Source: three-view drawing plus pictorial views. Frame: mm from the lowest corner of the part. A direction names the side the tool comes from. Round coordinates to 2 decimals unless told otherwise and drop trailing zeros. Order: outer loops, then holes, each group sorted by start corner. A loop starts at its lowest first (then second) coordinate and runs counter-clockwise, first axis right, second up. Notation, with made-up numbers: (28, -23.5) -> (47, -23.5) arc R28 cw to (47, 10.5) -> close; hole circle Ø2 at (-38.75, 33.25). An arc over 180 degrees is marked (long way). Answer as CSV lines item,"result".
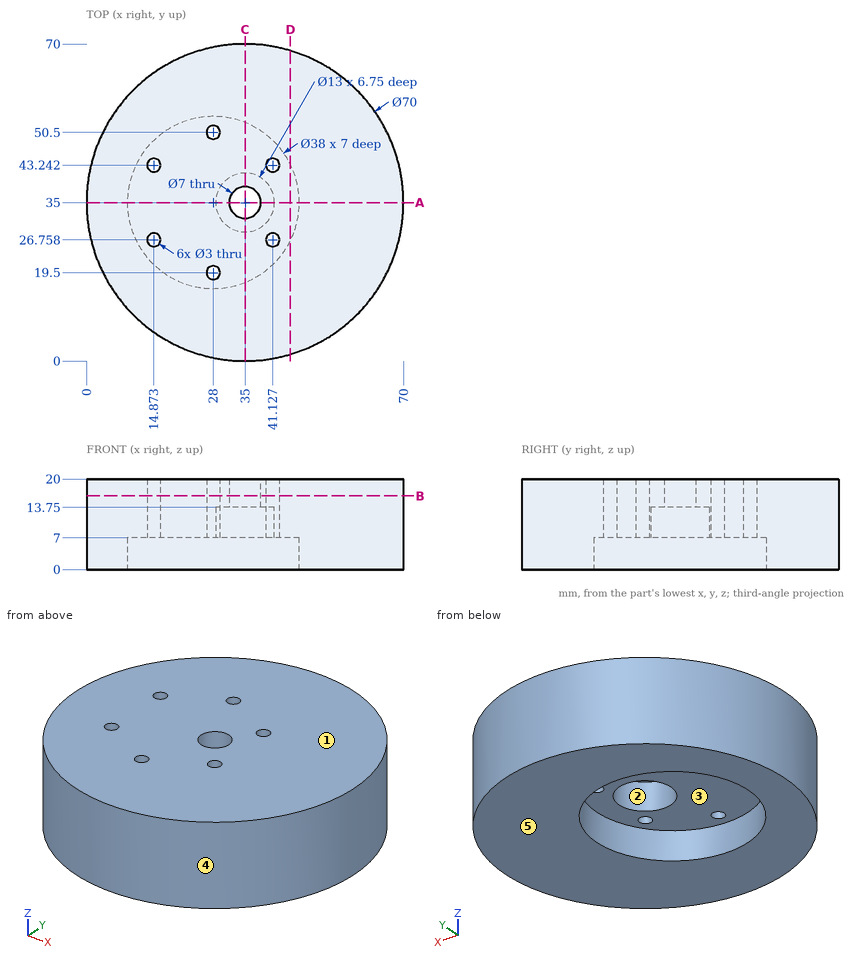
1. Pin query (flat end, axial travel): pin 1 (1.8 mm diameter, centred on x = 41.13, y = 43.24, fed in from -Z); pin 2 (1.5 mm diameter, centred on y = 43, z = 3, fed in from +X); pin 3 (12 mm diameter, centred on x = 48, z = 4, fed in from +Y); pin 4 (4 mm diameter, centred on y = 54.5, z = 5, fed in from -X). Return the tip coordinate at first contact, or that it passes through.
Results below:
pin 1,"through"
pin 2,"x = 69.24"
pin 3,"y = 69.29"
pin 4,"x = 4.69"
2. Section query D-D on x = 45. Return loops of the section in (y, z).
Results below:
outline,"(1.46, 0) -> (26.51, 0) -> (26.51, 7) -> (43.49, 7) -> (43.49, 0) -> (68.54, 0) -> (68.54, 20) -> (1.46, 20) -> close"
3. Line query: L1, parallel to Y at x = 28, z = 17; L2, parallel to Z at x = 35.5, y = 40; L3, parallel to Y at x = 41, z = 5.5. Output: solid intervals per line, ascending. Write a range as [from, to].
Results below:
L1,"[0.71, 18], [21, 49], [52, 69.29]"
L2,"[13.75, 20]"
L3,"[0.52, 21.14], [48.86, 69.48]"
4. Reachability of the marked faces 1 and 2 from +Z, -Z, +X, -X, +Y, -Y: full face, straight path, thin tool, end or side. Return the list, or none.
Results below:
face 1,"+Z, +X, -X, +Y, -Y"
face 2,"-Z"
5. Section query C-C on x = 35. Return loops of the section in (y, z).
Results below:
outline,"(0, 0) -> (17.34, 0) -> (17.34, 7) -> (28.5, 7) -> (28.5, 13.75) -> (31.5, 13.75) -> (31.5, 20) -> (0, 20) -> close; (38.5, 13.75) -> (41.5, 13.75) -> (41.5, 7) -> (52.66, 7) -> (52.66, 0) -> (70, 0) -> (70, 20) -> (38.5, 20) -> close"
6. Section query B-B on z = 16.25. Return loops of the section in (x, y), and give its area (3 significant figures).
Results below:
outline,"circle Ø70 at (35, 35); hole circle Ø3 at (14.87, 26.76); hole circle Ø3 at (14.87, 43.24); hole circle Ø3 at (28, 19.5); hole circle Ø3 at (28, 50.5); hole circle Ø7 at (35, 35); hole circle Ø3 at (41.13, 26.76); hole circle Ø3 at (41.13, 43.24)"
area,"3,770 mm2"
7. Mould query, pull axis X, two halves, no side actions, for the marked faces 3, 4 and 5. Classes: released by +X, released by -X, zero draft, split by the parting line, or undercut.
Results below:
face 3,"undercut"
face 4,"split by the parting line"
face 5,"zero draft"
8. Section query A-A on y = 35. Return loops of the section in (x, z).
Results below:
outline,"(0, 0) -> (9, 0) -> (9, 7) -> (28.5, 7) -> (28.5, 13.75) -> (31.5, 13.75) -> (31.5, 20) -> (0, 20) -> close; (38.5, 13.75) -> (41.5, 13.75) -> (41.5, 7) -> (47, 7) -> (47, 0) -> (70, 0) -> (70, 20) -> (38.5, 20) -> close"
